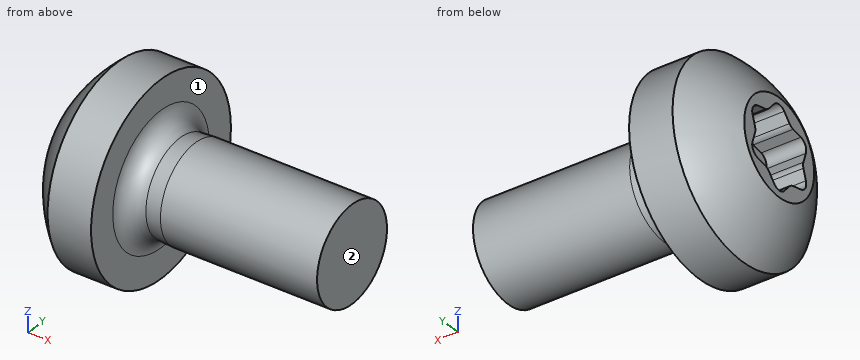
Autodesk Inventor part; units mm, degrees
ref_plane "YZ Plane" through (0, 0, 0) normal (1, 0, 0) x (0, 1, 0)
ref_plane "XZ Plane" through (0, 0, 0) normal (0, 1, 0) x (-1, 0, 0)
ref_plane "XY Plane" through (0, 0, 0) normal (0, 0, 1) x (1, 0, 0)
sketch "Sketch4" plane through (0, 0, 0) normal (0, 0, 1) x (1, 0, 0)
  line L0 (-2.1, 0) -> (5, 0)
  line L1 (0, 0) -> (-2.1, 0)
  line L2 (0, 2.5) -> (0, 1.725)
  line L3 (0.5, 1.225) -> (0.5, 1.225)
  line L4 (0.5, 1.225) -> (0.9, 1.25)
  arc A0 (0, 1.725) -> (0.5, 1.225) centre (0.5, 1.725) ccw
  line L5 (-2.1, 0) -> (-2.1, 1.25)
  line L6 (0, 2.5) -> (-1.1375, 2.5)
  arc A1 (-1.1375, 2.5) -> (-2.1, 1.25) centre (1.4883, -0.5175) ccw
  line L7 (0.9, 1.25) -> (5, 1.25)
  line L8 (5, 1.25) -> (5, 0)
  point P0 (0, 1.225)
  dimension "d71" = 0.5
  dimension "d72" = 5
  dimension "d74" = 0.4
  dimension "d75" = 2.45
  dimension "d78" = 2.5
  dimension "d82" = 4
  dimension "d83" = 2.1
  dimension "d84" = 5
  dimension "d104" = 4.1
  dimension "d105" = 2.5
revolve "Revolution7" add sketch "Sketch4" angle 360 about axis through (-2.1, 0, 0) along (1, 0, 0)
sketch "Sketch5" plane through (-2.1, 0, 0) normal (-1, 0, 0) x (0, 0, 1)
  circle A0 centre (0, 0) radius 1.2 construction
  circle A1 centre (0, 0) radius 0.84 construction
  line L0 (0, 0) -> (-0.7275, 0.42)
  line L1 (0, 0) -> (-0.7275, -0.42)
  line L2 (-1.8008, 0) -> (1.7887, 0)
  line L3 (-1.2, 0) -> (-0.7275, -0.42)
  line L4 (-1.2, 0) -> (-0.7275, 0.42)
  dimension "d88" = 2.4
  dimension "d89" = 1.68
  dimension "d90" = 30
  dimension "d91" = 30
extrude "Extrusion1" cut sketch "Sketch5" against normal blind 1.04
pattern_circular "Circular Pattern1" count 6 over 360 about axis through (-10, 0, 0) along (1, 0, 0) of "Extrusion1"
fillet "Fillet1" radius 0.24 12 edges at (-1.58, -1.0392, -0.6) (-1.58, -0.42, -0.7275) (-1.58, -0.84, 0) (-1.58, -1.0392, 0.6) (-1.58, -0.42, 0.7275) (-1.58, 0, 1.2) (-1.58, 0.84, 0) (-1.58, 1.0392, 0.6) (-1.58, 0.42, 0.7275) (-1.58, 0.42, -0.7275) (-1.58, 0, -1.2) (-1.58, 1.0392, -0.6)
thread "Thread7"
equation "\"a\" = 0.9"
equation "\"b\" = 4.1"
equation "\"dk\" = 5"
equation "\"k\" = 2.1"
equation "\"r\" = 0.5"
equation "\"rf\" = 4"
equation "\"x\" = 0.4"
equation "\"A_\" = 2.4"
equation "\"t\" = 1.04"
equation "\"p\" = 0.45"
equation "\"l_\" = 5"
equation "\"d\" = 2.5"
equation "\"ds_\" = 2.45"
equation "\"lg\" = 0"
properties part number "Flachkopfschraube mit Innenrund ISO 14583 - M2,5 x 5 - 4.8" material "Steel"
For this review, take the finished solid that the model builds, in its own axes (mm). Face numbers are marked on the shaded views. A direction names the side the tool comes from. Give positions to 0.01 mm unless a question says otherwise; leave off trailing zeros. Loops run counter-clockwise (first coordinate to the right, second up) from the corner with the lowest first, then second, coordinate; pieces in that order, holes last. Notation, with made-up numbers: M -31,-26.5 L 11,-26.5 A16 ccw 11,-1.5 Z; hole C -5,-34.75 d5. An arc over 180 degrees is marked long. Answer as a JSON object with one key per item and string values. Group by question number.
Q1. For probe 1 along Z at (x, y) = (-1.5, -0.75); probe 2 along X at (y, z) = (0.75, -0.2); probe 3 along Z at (x, y) = (3.5, -0.9), list the stretches that pass through material, from the lowest coordinate up. Write a range as [from, to].
Q2. Insertion check: P1, Ø1.5, axis at x = 0, y = 1.5, coming from the -Z side; P2, Ø2, axis at x = 4, z = 1.5, coming from the -Y side. Each pin has a flat end and moves straight along its axis. Give the tip position at first contact, or say it passes through.
Q3. Add section A-A on x = 2.75. Give the boundary of the cut face in (y, z).
Q4. Tool access review of the marked faces 1 and 2: name each direction out of +Z, -Z, +X, -X, +Y, -Y from which nothing blocks a thin tool from reaching the whole face with its end or side.
Checked values:
{
 "1": {"probe 1": "[-2.01, -0.66], [0.66, 2.01]", "probe 2": "[-1.06, 5]", "probe 3": "[-0.87, 0.87]"},
 "2": {"P1": "z = -2.38", "P2": "y = -1.15"},
 "3": {"outline": "C 0,0 d2.5"},
 "4": {"face 1": "+X", "face 2": "+Z, -Z, +X, +Y, -Y"}
}
